Autodesk Inventor part; units mm, degrees
ref_plane "YZ Plane" through (0, 0, 0) normal (1, 0, 0) x (0, 1, 0)
ref_plane "XZ Plane" through (0, 0, 0) normal (0, 1, 0) x (-1, 0, 0)
ref_plane "XY Plane" through (0, 0, 0) normal (0, 0, 1) x (1, 0, 0)
ref_plane "Arbeitsebene1" through (-0.0218, -0.0069, 0) normal (0, 0, 1) x (1, 0, 0)
sketch "Skizze1" plane through (-0.0218, -0.0069, 0) normal (0, 0, 1) x (1, 0, 0)
  circle A0 centre (-5.0753, -17.2861) radius 1.4
  circle A1 centre (-17.3974, -5.2209) radius 1.4
  arc A2 (5.7175, 26.2743) -> (7.9904, 25.6763) centre (6.0829, 23.0449) ccw
  arc A3 (5.7175, 26.2743) -> (-18.7943, -19.1862) centre (0.0218, 0.0069) ccw
  arc A4 (-18.1485, -19.7987) -> (-18.7943, -19.1862) centre (-16.256, -17.1565) ccw
  arc A5 (-18.1485, -19.7987) -> (25.9771, 6.988) centre (0.0218, 0.0069) ccw
  arc A6 (25.268, 9.2287) -> (25.9771, 6.988) centre (22.7337, 7.1941) ccw
  arc A7 (25.268, 9.2287) -> (7.9904, 25.6763) centre (0.0218, 0.0069) ccw
  spline S0 degree 3 poles (-11.5335, -6.2903) (-11.3493, -6.4745) (-11.2029, -6.6929) (-11.002, -7.1734) (-10.9495, -7.431) (-10.9461, -7.9517) (-10.9953, -8.2099) (-11.1865, -8.6846) (-11.3236, -8.8981) (-11.4967, -9.0805) knots 0 0 0 0 0.252225 0.252225 0.504373 0.504373 0.756494 0.756494 1 1 1 1
  line L0 (-11.5335, -6.2903) -> (-16.328, -1.4959)
  arc A8 (-16.328, 1.5053) -> (-16.328, -1.4959) centre (-14.8274, 0.0047) ccw
  line L1 (-16.328, 1.5053) -> (-1.4787, 16.3546)
  arc A9 (1.5225, 16.3546) -> (-1.4787, 16.3546) centre (0.0219, 14.854) ccw
  line L2 (1.5225, 16.3546) -> (16.3717, 1.5053)
  arc A10 (16.3717, -1.4959) -> (16.3717, 1.5053) centre (14.8711, 0.0047) ccw
  line L3 (16.3717, -1.4959) -> (1.5225, -16.3451)
  arc A11 (-1.4787, -16.3451) -> (1.5225, -16.3451) centre (0.0219, -14.8445) ccw
  line L4 (-1.4787, -16.3451) -> (-4.7731, -13.0507)
  spline S1 degree 3 poles (-7.5633, -13.0139) (-7.3743, -12.8347) (-7.1521, -12.694) (-6.6664, -12.5059) (-6.4076, -12.4602) (-5.8869, -12.4706) (-5.6301, -12.5266) (-5.1606, -12.7303) (-4.9509, -12.873) (-4.7731, -13.0507) knots 0 0 0 0 0.252231 0.252231 0.504388 0.504388 0.756517 0.756517 1 1 1 1
  arc A12 (-11.4967, -9.0805) -> (-7.5633, -13.0139) centre (-9.478, -10.9953) ccw
  line L5 (-17.3974, -5.2209) -> (-5.0753, -17.2861)
  line L6 (-17.8503, -0.0022) -> (0.0001, -17.8526)
  line L7 (0.0001, -17.8526) -> (-3.889, -21.7417)
  line L8 (-6.7174, -21.7417) -> (-21.7394, -6.7197)
  line L9 (-21.7394, -3.8912) -> (-17.8503, -0.0022)
  arc A13 (-21.7394, -3.8912) -> (-21.7394, -6.7197) centre (-20.3252, -5.3055) ccw
  arc A14 (-6.7174, -21.7417) -> (-3.889, -21.7417) centre (-5.3032, -20.3275) ccw
  line L10 (-17.8503, -0.0022) -> (-18.5575, -0.7093)
  line L11 (-15.729, -0.7093) -> (-0.707, -15.7313)
  line L12 (-0.707, -18.5597) -> (0.0001, -17.8526)
  line L13 (0.0001, -17.8526) -> (-17.8503, -0.0022)
  arc A15 (-15.729, -0.7093) -> (-18.5575, -0.7093) centre (-17.1432, -2.1235) ccw
  arc A16 (-0.707, -18.5597) -> (-0.707, -15.7313) centre (-2.1212, -17.1455) ccw
  circle A17 centre (5.2496, -17.4123) radius 1.4
  circle A18 centre (17.3147, -5.0902) radius 1.4
  point P0 (0.0218, 0.0069)
  point P1 (-5.3032, -23.1559)
  point P2 (-11.5553, -6.2972)
  point P3 (-16.3497, -1.5028)
  point P4 (-1.5005, -16.352)
  point P5 (-4.7949, -13.0576)
  point P6 (-17.1432, 0.705)
  dimension "d0" = 7.5
  dimension "d1" = 2
  dimension "d23" = 1
  dimension "d24" = 2
extrude "Extrusion1" add sketch "Skizze1" along normal blind 50 contours L0 A8 A15 L11 A16 A11 L4 S1 L6 S0 | S0 L6 A15 A8 L0 | L6 S1 A12 L5 S0 | S0 A12 S1 L6 A16 L7 A14 L8 A13 L9 A15 | S1 L4 A11 A16 L6 | L5 A12
sketch "Skizze2" plane through (-0.0218, -0.0069, 50) normal (0, 0, 1) x (1, 0, 0)
  line L0 (-21.1915, 0.0069) -> (0.0218, -21.2063)
  line L1 (-18.5575, -0.7093) -> (-21.7394, -3.8912)
  arc A0 (-21.7394, -3.8912) -> (-21.7394, -6.7197) centre (-20.3252, -5.3055) ccw
  line L2 (-21.7394, -6.7197) -> (-6.7174, -21.7417)
  arc A1 (-6.7174, -21.7417) -> (-3.889, -21.7417) centre (-5.3032, -20.3275) ccw
  line L3 (-3.889, -21.7417) -> (-0.707, -18.5597)
  circle A2 centre (-17.3974, -5.2209) radius 1.4
  circle A3 centre (-5.0753, -17.2861) radius 1.4
  arc A4 (-0.707, -18.5597) -> (-0.707, -15.7313) centre (-2.1212, -17.1455) ccw
  line L4 (-0.707, -15.7313) -> (-15.729, -0.7093)
  arc A5 (-15.729, -0.7093) -> (-18.5575, -0.7093) centre (-17.1432, -2.1235) ccw
  point P0 (0.0218, 0.0069)
  point P1 (-1.6659, -19.5187)
  point P2 (-3.6908, -17.4938)
  point P3 (-5.283, -15.9016)
  point P4 (-15.9978, -5.1867)
  point P5 (-17.3632, -3.8213)
  point P6 (-19.5164, -1.6682)
extrude "Extrusion2" add sketch "Skizze2" along normal blind 4 contours L0 A2 A3 L3 A1 L2 A0 L1
sketch "Skizze3" plane through (-0.0218, -0.0069, 54) normal (0, 0, 1) x (1, 0, 0)
  line L0 (21.2132, 0) -> (0, 21.2132)
  line L1 (0, 21.2132) -> (-21.2132, 0)
  line L2 (-21.2132, 0) -> (0, -21.2132)
  line L3 (0, -21.2132) -> (21.2132, 0)
  circle A0 centre (0, 0) radius 1.3301
  circle A1 centre (-10.6066, 0) radius 1.5
  circle A2 centre (0, -10.6066) radius 1.5
  circle A3 centre (10.6066, 0) radius 1.5
  circle A4 centre (0, 10.6066) radius 1.5
  line L4 (-3.889, -21.7417) -> (-1.6659, -19.5187)
  line L5 (-1.6659, -19.5187) -> (-3.6908, -17.4938)
  arc A5 (-5.283, -15.9016) -> (-3.6908, -17.4938) centre (-5.0753, -17.2861) ccw
  line L6 (-5.283, -15.9016) -> (-15.9978, -5.1867)
  arc A6 (-17.3632, -3.8213) -> (-15.9978, -5.1867) centre (-17.3974, -5.2209) ccw
  line L7 (-17.3632, -3.8213) -> (-19.5164, -1.6682)
  line L8 (-19.5164, -1.6682) -> (-21.7394, -3.8912)
  arc A7 (-21.7394, -3.8912) -> (-21.7394, -6.7197) centre (-20.3252, -5.3055) ccw
  line L9 (-21.7394, -6.7197) -> (-6.7174, -21.7417)
  arc A8 (-6.7174, -21.7417) -> (-3.889, -21.7417) centre (-5.3032, -20.3275) ccw
  arc A9 (-15.9978, -5.1867) -> (-17.3632, -3.8213) centre (-17.3974, -5.2209) ccw
  arc A10 (-3.6908, -17.4938) -> (-5.283, -15.9016) centre (-5.0753, -17.2861) ccw
  circle A11 centre (-10.6066, 0) radius 1.4
  circle A12 centre (0, 10.6066) radius 1.4
  circle A13 centre (10.6066, 0) radius 1.4
  circle A14 centre (0, -10.6066) radius 1.4
  line L10 (-19.5164, -1.6682) -> (1.6825, 19.5307)
  line L11 (-1.6659, -19.5187) -> (19.533, 1.6802)
  point P0 (0.0218, 0.0069)
  point P1 (-19.5307, -1.6825)
  point P2 (-1.6802, -19.533)
  dimension "d14" = 2.8
  dimension "d15" = 2.8
  dimension "d16" = 2.8
  dimension "d17" = 2.8
extrude "Extrusion3" add sketch "Skizze3" along normal blind 4 contours L11 L5 A10 L6 A9 L7 L10 L0 | L4 L2 A5 L5 | L4 A8 L9 A7 L8 L2 A6 A5 | L7 A6 L2 L8 | A5 L2 A6 L6 | A1 | A2 | A3 | A4
sketch "Skizze4" plane through (-0.0073, -17.8452, 50) normal (0.7071068, -0.7071068, 0) x (-0.7071068, -0.7071068, 0)
  line L0 (5.5202, 50) -> (1.0202, 50)
  line L1 (2.3764, 0) -> (1.0202, 0)
  line L2 (2.3764, 0) -> (2.3764, -4)
  line L3 (5.5202, -8) -> (-27.6034, -8)
  line L4 (5.5202, 50) -> (5.5202, -8)
  line L5 (-2.5, 9.2593) -> (2.5, 9.2593)
  line L6 (2.5, 9.2593) -> (2.5, 12.2593)
  line L7 (2.5, 12.2593) -> (-2.5, 12.2593)
  line L8 (-2.5, 12.2593) -> (-2.5, 9.2593)
  line L9 (-2.5, 9.2593) -> (2.5, 12.2593) construction
  line L10 (2.5, 9.2593) -> (-2.5, 12.2593) construction
  line L11 (0, 9.2593) -> (2.5, 7.8159)
  line L12 (0, 9.2593) -> (2.8868, 9.2593) construction
  line L13 (2.5, 7.8159) -> (2.5, 13.7027)
  line L14 (2.5, 13.7027) -> (0, 12.2593)
  line L15 (2.3764, -4) -> (-27.6034, -4)
  line L16 (-27.6034, -4) -> (-27.6034, -8)
  line L17 (1.0202, 50) -> (1.0202, 0)
  point P0 (-12.6236, 50)
  point P1 (0, 10.7593)
  point P2 (2.5, 9.2593)
  dimension "d8" = 5
  dimension "d9" = 3
  dimension "d10" = 30
  dimension "d11" = 30
extrude "Extrusion4" cut sketch "Skizze4" against normal through all contours L7 L17 L5 L8 | L7 L6 L5 L17 | L17 L11 L5 | L5 L13 L11 L17
sketch "Skizze5" plane through (-0.0218, -0.0069, 58) normal (0, 0, 1) x (1, 0, 0)
  circle A0 centre (-17.3974, -5.2209) radius 1.4
  circle A1 centre (-5.0753, -17.2861) radius 1.4
  circle A2 centre (-17.3974, -5.2209) radius 3.25
  circle A3 centre (-5.0753, -17.2861) radius 3.25
  point P0 (0.0218, 0.0069)
  dimension "d19" = 6.5
  dimension "d20" = 6.5
extrude "Extrusion5" cut sketch "Skizze5" against normal blind 30 contours A0 | A1 | A2 | A3
sketch "Skizze6" plane through (-3.9107, -21.7486, 58) normal (0.7071068, -0.7071068, 0) x (-0.7071068, -0.7071068, 0)
  line L0 (0.9383, 30) -> (-5.5617, 30)
  line L1 (-14.2171, 61.056) -> (6.1145, 61.056)
  line L2 (6.1145, 61.056) -> (6.1145, 38)
  line L3 (6.1145, 38) -> (-14.2171, 38)
  line L4 (-14.2171, 38) -> (-14.2171, 61.056)
  line L5 (0, 58) -> (-4.5, 58)
  point P0 (-18.1439, 58)
  dimension "d25" = 20
extrude "Extrusion6" cut sketch "Skizze6" against normal blind 50
properties part number "IM_ledmatrix_holder"
For this review, take the finished solid that the model builds, in its own axes (mm). A direction names the side the tool comes from. Coordinates: 2 decimals unless noted, no trailing zeros. Write each loop counter-clockwise with the first axis right and the second up, starting at its lowest first coordinate (ties: lowest second). Pieces come first, ordered by that corner, then holes. Notation, with made-up numbers: (48.25, 74) - (106.25, 74) arc R18 ccw to (106.25, 95) - close; hole circle Ø4 at (-25.5, 39). An arc over 180 degrees is marked (long way). Answer in a Markdown table with one row per item. Add a question column.
Q1. For probe 1 along Z at (x, y) = (7, 5); probe 2 along Y at (x, z) = (-19, 48); probe 3 along Y at (x, z) = (-7, 44), list the stretches that pass through material, from the lowest coordinate up.
Q2. For P1, Ø5, axis at y = -12.5, z = 38.5, coming from the +X side; P2, Ø1.7, axis at x = -10.63, y = -0.01, coming from the -Z side; P3, Ø12, axis at x = -16, z = 34, coming from the +Y side; P4, Ø2, axis at x = -4.5, y = -1, coming from the -Z side, all flat-tipped, find the tip position at first contact; note any pin that passes through.
Q3. We need section B-B, the plane z = 23.5. State the section outline as (x, y) points (3 decimals).
Q4. Tool access review of faces 1 (the flat face through (-8.345, -8.122, 45.306)), 2 (the cylindrical face through (-0.143, -17.13, 28.746)), 3 (the cylindrical face through (-17.19, -0.13, 28.75)), 4 (the cylindrical face through (-7.676, -19.271, 43.21)), 5 (the flat face through (-9, -9, 37.741)): name each direction out of +Z, -Z, +X, -X, +Y, -Y from which nothing blocks a thin tool from reaching the whole face with its end or side.
Q5. We need section D-D, the plane x = -13.5. State the section outline as (y, z) points.
Q6. Draft analysis for pull direction Z (two halves, no side actions). For faces 6 (the cylindrical face through (-0.2, 9.21, 55.97)), 7 (the flat face through (-10.66, -10.73, 39.99)), 8 (the flat face through (-3.7, -18, 28)), state which applies: +Z half, -Z half, draft (parallel to the pull), parting line (faces both ways), or undercut.
Q7. We need section A-A, the plane x = 0.5. State the section outline as (y, z) points.
Answer list:
| question | item | result |
|---|---|---|
| 1 | probe 1 | z = 54 to 58 |
| 1 | probe 2 | y = -9.49 to -8.07, -2.39 to -1.14 |
| 1 | probe 3 | y = -21.49 to -19.93, -14.66 to -9.47 |
| 2 | P1 | stops at x = -1.59 |
| 2 | P2 | passes through |
| 2 | P3 | stops at y = -0.13 |
| 2 | P4 | stops at z = 54 |
| 3 | outline | (-21.761, -6.727) - (-6.739, -21.749) arc R2 ccw to (-3.911, -21.749) - (-0.729, -18.567) arc R2 ccw to (-0.729, -15.738) - (-15.751, -0.716) arc R2 ccw to (-18.579, -0.716) - (-21.761, -3.898) arc R2 ccw to start; hole circle Ø2.8 at (-17.419, -5.228); hole circle Ø2.8 at (-5.097, -17.293) |
| 4 | face 1 | -Z, +X, +Y |
| 4 | face 2 | -Z, +X |
| 4 | face 3 | -Z, +Y |
| 4 | face 4 | +Z |
| 4 | face 5 | +X, +Y |
| 5 | outline | (-14.99, 20) - (-2.97, 20) - (-2.97, 37.74) - (-7.89, 37.74) - (-7.89, 42.18) - (-4.35, 40.74) - (-2.97, 40.74) - (-2.97, 50) - (-7.71, 50) - (-7.71, 54) - (4.36, 54) - (4.36, 58) - (-14.99, 58) - close |
| 6 | face 6 | draft |
| 6 | face 7 | undercut |
| 6 | face 8 | +Z half |
| 7 | outline | (-17.34, 54) - (-11.91, 54) - (-11.91, 58) - (-17.34, 58) - close; (-9.31, 54) - (-1.23, 54) - (-1.23, 58) - (-9.31, 58) - close; (1.22, 54) - (9.3, 54) - (9.3, 58) - (1.22, 58) - close; (11.9, 54) - (18.36, 54) - (18.36, 58) - (11.9, 58) - close |
